Autodesk Inventor part; units mm, degrees
ref_plane "YZ Plane" through (0, 0, 0) normal (1, 0, 0) x (0, 1, 0)
ref_plane "XZ Plane" through (0, 0, 0) normal (0, 1, 0) x (-1, 0, 0)
ref_plane "XY Plane" through (0, 0, 0) normal (0, 0, 1) x (1, 0, 0)
sketch "Sketch1" plane through (0, 0, 0) normal (0, 1, 0) x (-1, 0, 0)
  line L0 (33.5, 64.5) -> (-33.5, 64.5)
  line L1 (-33.5, 64.5) -> (-33.5, -64.5)
  line L2 (-33.5, -64.5) -> (33.5, -64.5)
  line L3 (33.5, -64.5) -> (33.5, 64.5)
  line L4 (33.5, 64.5) -> (-33.5, -64.5) construction
  line L5 (-33.5, 64.5) -> (33.5, -64.5) construction
  point P0 (0, 0)
  dimension "d0" = 67
  dimension "d1" = 129
extrude "Extrusion1" add sketch "Sketch1" along normal blind 3
sketch "Sketch2" plane through (0, 0, 0) normal (0, -1, 0) x (1, 0, 0)
  circle A0 centre (0, 51.5) radius 3
  line L0 (-2, 39.5) -> (-2, 37.5)
  line L1 (2, 37.5) -> (2, 39.5)
  circle A1 centre (0, 8.5) radius 3.487
  circle A2 centre (0, -21.5) radius 2
  circle A3 centre (0, -33.5) radius 3
  arc A4 (2, 39.5) -> (-2, 39.5) centre (0, 39.5) ccw
  arc A5 (-2, 37.5) -> (2, 37.5) centre (0, 37.5) ccw
  line L2 (-33.5, 64.5) -> (33.5, 64.5)
  point P0 (0, 0)
  point P1 (2, 38.5)
  point P2 (-2, 38.5)
  dimension "d4" = 6
  dimension "d7" = 4
  dimension "d8" = 6
  dimension "d9" = 13
  dimension "d10" = 56
  dimension "d11" = 26
  dimension "d12" = 60
  dimension "d13" = 85
hole "Hole1" at (0, 0, 51.5) at (0, 0, -33.5) direction (0, 1, 0) diameter 4.917 depth 17.1
hole "Hole2" at (0, 0, -21.5) at (0, 0, 39.5) at (0, 0, 37.5) direction (0, 1, 0) diameter 4 depth 17.1
hole "Hole3" at (0, 0, 8.5) direction (0, 1, 0) diameter 4.9784 depth 19.05
sketch "Sketch3" plane through (-33.5, 0, 64.5) normal (0, 0, 1) x (1, 0, 0)
  line L0 (0, 3) -> (67, 3)
  line L1 (0, 3) -> (67, 3)
  line L2 (67, 3) -> (67, 0)
  line L3 (67, 0) -> (0, 0)
  line L4 (0, 0) -> (0, 3)
  point P0 (33.5, 0)
extrude "Extrusion2" add sketch "Sketch3" along normal blind 3
sketch "Sketch4" plane through (0, 3, 0) normal (0, 1, 0) x (1, 0, 0)
  line L0 (-33.5, 64.5) -> (-33.5, -67.5)
  line L1 (33.5, 64.5) -> (33.5, -67.5)
  line L2 (-33.5, -67.5) -> (33.5, -67.5)
  line L3 (33.5, -67.5) -> (33.5, -64.5)
  line L4 (33.5, -64.5) -> (-33.5, -64.5)
  line L5 (-33.5, -64.5) -> (-33.5, -67.5)
  point P0 (0, 0)
  point P1 (-33.5, -64.5)
  dimension "d37" = 3
extrude "Extrusion3" add sketch "Sketch4" along normal blind 45
sketch "Sketch5" plane through (-33.5, 0, 67.5) normal (0, 0, 1) x (1, 0, 0)
  circle A0 centre (33.5, 23.5) radius 20.5
  line L0 (0, 0) -> (67, 0)
  line L1 (0, 48) -> (67, 48)
  point P0 (33.5, 0)
  point P1 (33.5, 48)
  dimension "d40" = 41
  dimension "d41" = 23.5
extrude "Extrusion4" cut sketch "Sketch5" against normal blind 45
sketch "Sketch6" plane through (-33.5, 0, -64.5) normal (-1, 0, 0) x (0, 0, 1)
  line L0 (0, 0) -> (0, 3)
  line L1 (132, 0) -> (0, 0)
  line L2 (0, 3) -> (132, 3)
  line L3 (132, 3) -> (132, 0)
  line L4 (132, 0) -> (0, 0)
  line L5 (0, 0) -> (0, 3)
  point P0 (64.5, 0)
extrude "Extrusion5" add sketch "Sketch6" along normal blind 5
sketch "Sketch7" plane through (0, 3, 0) normal (0, 1, 0) x (1, 0, 0)
  line L0 (33.5, -67.5) -> (-38.5, -67.5)
  line L1 (33.5, 64.5) -> (-38.5, 64.5)
  line L2 (-38.5, -67.5) -> (-33.5, -67.5)
  line L3 (-33.5, -67.5) -> (-33.5, 64.5)
  line L4 (-33.5, 64.5) -> (-38.5, 64.5)
  line L5 (-38.5, 64.5) -> (-38.5, -67.5)
  point P0 (0, 0)
  point P1 (-38.5, 64.5)
  dimension "d46" = 5
extrude "Extrusion6" add sketch "Sketch7" along normal blind 45
sketch "Sketch8" plane through (33.5, 0, -64.5) normal (0, 0, -1) x (-1, 0, 0)
  line L0 (0, 48) -> (67, 48)
  line L1 (72, 0) -> (72, 48)
  line L2 (67, 48) -> (72, 48)
  line L3 (72, 48) -> (72, 0)
  line L4 (72, 0) -> (67, 0)
  line L5 (67, 0) -> (67, 48)
  point P0 (33.5, 0)
extrude "Extrusion7" add sketch "Sketch8" along normal blind 14
sketch "Sketch9" plane through (-33.5, 0, 67.5) normal (0, 0, 1) x (1, 0, 0)
  line L0 (-5, 0) -> (-5, 48)
  line L1 (67, 0) -> (-5, 0)
  line L2 (-5, 48) -> (0, 48)
  line L3 (0, 48) -> (0, 0)
  line L4 (0, 0) -> (-5, 0)
  line L5 (-5, 0) -> (-5, 48)
  point P0 (33.5, 0)
  dimension "d51" = 5
extrude "Extrusion8" add sketch "Sketch9" along normal blind 14
sketch "Sketch10" plane through (0, 0, 0) normal (0, -1, 0) x (1, 0, 0)
  line L0 (-33.5, 64.5) -> (-33.5, -78.5)
  line L1 (-38.5, 81.5) -> (-33.5, 81.5)
  line L2 (-33.5, -78.5) -> (-38.5, -78.5)
  line L3 (-38.5, -78.5) -> (-38.5, 81.5)
  line L4 (-38.5, 81.5) -> (-33.5, 81.5)
  line L5 (-33.5, 81.5) -> (-33.5, -78.5)
  point P0 (0, 0)
sketch "Sketch11" plane through (-33.5, 3, 64.5) normal (1, 0, 0) x (0, 0, -1)
  circle A0 centre (136, 9.75) radius 2
  circle A1 centre (135.5136, 34.75) radius 2
  line L0 (143, -5) -> (-17, -5)
  line L1 (143, 45) -> (143, -3)
  circle A2 centre (-10, 9.75) radius 2
  circle A3 centre (-10, 34.75) radius 2
  line L2 (-17, 45) -> (-17, -5)
  point P0 (64.5, -3)
  dimension "d56" = 4
  dimension "d57" = 4
  dimension "d58" = 14.75
  dimension "d59" = 7
  dimension "d60" = 25
  dimension "d68" = 4
  dimension "d69" = 14.75
  dimension "d70" = 7
  dimension "d71" = 7
  dimension "d72" = 25
hole "Hole4" at (-33.5, 37.75, -71.0136) at (-33.5, 12.75, -71.5) at (-33.5, 37.75, 74.5) at (-33.5, 12.75, 74.5) direction (-1, 0, 0) diameter 3.242 depth 10 tip angle 118
sketch "Sketch12" plane through (-33.5, 3, 64.5) normal (1, 0, 0) x (0, 0, -1)
  line L0 (-3, 45) -> (0, 45)
  line L1 (0, 45) -> (129, 45)
  line L2 (129, 45) -> (129, 41)
  line L3 (129, 41) -> (0, 41)
  line L4 (0, 41) -> (0, 45)
  point P0 (64.5, -3)
  dimension "d73" = 129
  dimension "d74" = 4
extrude "Extrusion10" add sketch "Sketch12" along normal up to surface (67 mm away)
hole "Hole5" at (0, 0, 51.5) at (0, 0, -33.5) direction (0, 1, 0) diameter 4.917 end through all
hole "Hole6" at (0, 0, 8.5) direction (0, 1, 0) diameter 4.9784 end through all
hole "Hole7" at (0, 0, -21.5) at (0, 0, 39.5) at (0, 0, 37.5) direction (0, 1, 0) diameter 4 end through all
sketch "Sketch13" plane through (0, 3, 0) normal (0, 1, 0) x (1, 0, 0)
  line L0 (-33.5, 64.5) -> (-33.5, -64.5)
  line L1 (33.5, 64.5) -> (-33.5, 64.5)
  line L2 (-33.5, -64.5) -> (33.5, -64.5)
  line L3 (33.5, -64.5) -> (33.5, 64.5)
  line L4 (33.5, 64.5) -> (-33.5, 64.5)
  line L5 (-33.5, 64.5) -> (-33.5, -64.5)
  point P0 (0, 0)
extrude "Extrusion11" cut sketch "Sketch13" against normal blind 10
sketch "Sketch14" plane through (0, 0, 0) normal (0, -1, 0) x (1, 0, 0)
  line L0 (58.5292, 135.8199) -> (-75.2061, 135.8199)
  line L1 (-75.2061, 135.8199) -> (-75.2061, -131.0093)
  line L2 (-75.2061, -131.0093) -> (58.5292, -131.0093)
  line L3 (58.5292, -131.0093) -> (58.5292, 135.8199)
  point P0 (0, 0)
extrude "Extrusion12" cut sketch "Sketch14" against normal blind 2
properties part number "Laser Bracket"
The model under review builds one solid part; all positions refer to its coordinate system, in mm. A direction names the side the tool comes from. Coordinates: 2 decimals unless noted, no trailing zeros. Write each loop counter-clockwise with the first axis right and the second up, starting at its lowest first coordinate (ties: lowest second). Pieces come first, ordered by that corner, then holes.
1) We need section B-B on y = 8. State the section outline as (x, z) points, then the cut area to 4 significant figures.
2) The part is to be moulded in two halves that separate along Z. For faces 1 (the face through (-36.035, 37.679, -69.394)), 2 (the face through (-38.5, 25, 0)), 3 (the face through (-36.035, 38.371, 73.003)), 4 (the face through (-36, 25, -78.5)), say which applies: pulls with the +Z half, pulls with the -Z half, needs draft (parallel to the pull), parting line crosses it, or undercut.
3) To check wall thickness, follow probe 1 along Z at (x, y) = (-35.85, 37.75); probe 2 along Z at (x, y) = (0, 46.8); probe 3 along Z at (x, y) = (-35.3, 12.75). State the ranges of each line that lie inside material, in increasing order.
4) We need section A-A on z = 74.5. State the section outline as (x, y) points.
5) Clearance check with flat-ended pins moving along their axes: pin 1 Ø5 at (x, y) = (-21.5, 17) entering from -Z; pin 2 Ø2.5 at (x, z) = (0, -21.5) entering from -Y; pin 3 Ø14 at (y, z) = (23.5, 1) entering from +X; pin 4 Ø20 at (x, z) = (-4.5, -15.5) entering from -Y. State where each tip first meets the part, or that it passes through.
6) Machinability: for faces 5 (the face through (-0.06, 46.03, 41.5)), 6 (the face through (8, 4, 64.5)), 7 (the face through (0, 45, 67.5)), which of the approach directions +Z, -Z, +X, -X, +Y, -Y give a long, thin tool a straight path to every point of the face, cutting with its end or side? Answer none if there is none.
7) We need section C-C on z = 8.5. State the section outline as (x, y) points.
8) We need section D-D on x = 7. State the section outline as (y, z) points, then the cut area to 3 significant figures.
Answer list:
1. outline: (-38.5, -78.5) - (-33.5, -78.5) - (-33.5, 64.5) - (-13.42, 64.5) - (-13.42, 67.5) - (-33.5, 67.5) - (-33.5, 81.5) - (-38.5, 81.5) - close; (13.42, 64.5) - (33.5, 64.5) - (33.5, 67.5) - (13.42, 67.5) - close
1. area: 920.5 mm2
2. face 1: undercut
2. face 2: needs draft
2. face 3: undercut
2. face 4: pulls with the -Z half
3. probe 1: z = -78.5 to -72.63, -69.39 to 72.88, 76.12 to 81.5
3. probe 2: z = -64.5 to -35.96, -31.04 to -23.5, -19.5 to 6.01, 10.99 to 35.5, 41.5 to 49.04, 53.96 to 67.5
3. probe 3: z = -78.5 to -73.12, -69.88 to 72.88, 76.12 to 81.5
4. outline: (-38.5, 2) - (-33.5, 2) - (-33.5, 11.13) - (-38.5, 11.13) - close; (-38.5, 14.37) - (-33.5, 14.37) - (-33.5, 36.13) - (-38.5, 36.13) - close; (-38.5, 39.37) - (-33.5, 39.37) - (-33.5, 48) - (-38.5, 48) - close
5. pin 1: stops at z = 64.5
5. pin 2: passes through
5. pin 3: stops at x = -33.5
5. pin 4: stops at y = 44
6. face 5: +Y, -Y
6. face 6: -Z, +X, -Y
6. face 7: +Z, +X, +Y, -Y
7. outline: (-38.5, 2) - (-33.5, 2) - (-33.5, 44) - (-2.49, 44) - (-2.49, 48) - (-38.5, 48) - close; (2.49, 44) - (33.5, 44) - (33.5, 48) - (2.49, 48) - close
8. outline: (2, 64.5) - (4.23, 64.5) - (4.23, 67.5) - (2, 67.5) - close; (42.77, 64.5) - (44, 64.5) - (44, -64.5) - (48, -64.5) - (48, 67.5) - (42.77, 67.5) - close
8. area: 538 mm2
